Source: CAD feature listing. Evaluate the final solid. Frame: model axes, mm. A direction names the side the tool comes from. Give positions to 0.01 mm unless a question says otherwise; leave off trailing zeros. Write each loop counter-clockwise with the first axis right and the second up, starting at its lowest first coordinate (ties: lowest second). Pieces come first, ordered by that corner, then holes. Notation, with made-up numbers: M -20.75,36.5 L 38.25,36.5 A30 cw 38.25,71.5 Z; hole C -9.75,69 d10. An arc over 180 degrees is marked long. Answer as a JSON object with one key per item and string values. Group by question number.
```python
from build123d import *

# Parameters (mm, degrees)
SKETCH1_R           = 1.6
BOSS_EXTRUDE1_DEPTH = 2.5
SKETCH2_W           = 66
SKETCH2_H           = 2.5
BOSS_EXTRUDE2_DEPTH = 43
SKETCH3_W           = 5
SKETCH3_H           = 32.5
CUT_EXTRUDE1_DEPTH  = 9.5
LPATTERN1_COUNT     = 6
LPATTERN1_PITCH     = 10
SKETCH4_W           = 4
SKETCH4_H           = 15
CUT_EXTRUDE2_DEPTH  = 44
LPATTERN2_COUNT     = 5
LPATTERN2_PITCH     = 8


with BuildPart() as part:
    # Sketch1 → Boss-Extrude1 (new body)
    with BuildSketch(Plane(origin=(0, 0, 0), x_dir=(1, 0, 0), z_dir=(0, 1, 0))):
        Polygon((-33, 6), (-33, 16), (33, 16), (33, 6), (33, -6), (-33, -6), align=None)
        with Locations((-26, 11)):
            Circle(SKETCH1_R, mode=Mode.SUBTRACT)
        with Locations((-14.5, 11)):
            Circle(SKETCH1_R, mode=Mode.SUBTRACT)
    extrude(amount=BOSS_EXTRUDE1_DEPTH)

    # Sketch2 → Boss-Extrude2 (add)
    with BuildSketch(Plane(origin=(0, 0, 0), x_dir=(1, 0, 0), z_dir=(0, 1, 0))):
        with Locations((0, -7.25)):
            Rectangle(SKETCH2_W, SKETCH2_H)
    extrude(amount=BOSS_EXTRUDE2_DEPTH)

    # Sketch3 → Cut-Extrude1 (cut, through all)
    with BuildSketch(Plane.XY):
        with Locations((25.5, 22.75)):
            Rectangle(SKETCH3_W, SKETCH3_H)
    cut_extrude1 = extrude(amount=CUT_EXTRUDE1_DEPTH, mode=Mode.SUBTRACT)

    # LPattern1: Cut-Extrude1 ×6
    with Locations(*[(-i * LPATTERN1_PITCH, 0, 0) for i in range(1, LPATTERN1_COUNT)]):
        add(cut_extrude1, mode=Mode.SUBTRACT)

    # Sketch4 → Cut-Extrude2 (cut, through all)
    with BuildSketch(Plane(origin=(0, 0, 0), x_dir=(1, 0, 0), z_dir=(0, 1, 0))):
        with Locations((26, 5)):
            Rectangle(SKETCH4_W, SKETCH4_H)
    cut_extrude2 = extrude(amount=CUT_EXTRUDE2_DEPTH, mode=Mode.SUBTRACT)

    # LPattern2: Cut-Extrude2 ×5
    with Locations(*[(-i * LPATTERN2_PITCH, 0, 0) for i in range(1, LPATTERN2_COUNT)]):
        add(cut_extrude2, mode=Mode.SUBTRACT)


solid = part.part
```
(1) Section D-D, the plane z = -6. Return loops of the section in (x, y), plus the area to 3 significant figures.
(2) Ray query, L1, parallel to Z at x = -26, y = 0.9; L2, parallel to Y at x = 22, z = 3.25; L3, parallel to Z at x = 1, y = 9. Return the intervals inside material, ascending. Write a range as [from, to].
(3) Pull-direction query (Y, two-part tool) for faces 1 (the flat face through (2, 1, -12.5)), 2 (the flat face through (-0.5, 0, -3.9)), 3 (the flat face through (7.8, 2.5, -5.2)), 4 (the flat face through (28, 23, 7)); classes: pulls with the +Y half, pulls with the -Y half, needs draft (parallel to the pull), parting line crosses it, or undercut.
(4) Contact query for a flat-ended pin moving along its axis: pin 1 Ø12 at (x, z) = (8, -10) entering from +Y. Output: stop coordinate, or through.
(5) Section B-B, the plane y = 17. Return loops of the section in (x, z).
(6) Section C-C, the plane x = -14.5. Return loops of the section in (y, z).
(7) Access query for faces 5 (the flat face through (-33, 15, 6.3)), 6 (the flat face through (25, 39, 7)), 7 (the flat face through (10, 1, -12.5)). Directions: +Z, -Z, +X, -X, +Y, -Y. A direction counts if a zero-diameter tool reaches every point of the face in a straight line with its end or side. Return the directions, or none.
(8) Section A-A, the plane z = -11. State how many separate pieces and enclosed holes the cut face has, plus the area to 3 significant figures.
Reported:
{
 "1": {"outline": "M -33,0 L -8,0 L -8,2.5 L -33,2.5 Z; M -4,0 L 0,0 L 0,2.5 L -4,2.5 Z; M 4,0 L 8,0 L 8,2.5 L 4,2.5 Z; M 12,0 L 16,0 L 16,2.5 L 12,2.5 Z; M 20,0 L 24,0 L 24,2.5 L 20,2.5 Z; M 28,0 L 33,0 L 33,2.5 L 28,2.5 Z", "area": "115 mm2"},
 "2": {"L1": "z = [-16, -12.6], [-9.4, 8.5]", "L2": "y = [0, 2.5]", "L3": "z = [6, 8.5]"},
 "3": {"face 1": "needs draft", "face 2": "pulls with the -Y half", "face 3": "pulls with the +Y half", "face 4": "undercut"},
 "4": {"pin 1": "stops at y = 2.5"},
 "5": {"outline": "M -33,6 L -27,6 L -27,8.5 L -33,8.5 Z; M -22,6 L -17,6 L -17,8.5 L -22,8.5 Z; M -12,6 L -7,6 L -7,8.5 L -12,8.5 Z; M -2,6 L 3,6 L 3,8.5 L -2,8.5 Z; M 8,6 L 13,6 L 13,8.5 L 8,8.5 Z; M 18,6 L 23,6 L 23,8.5 L 18,8.5 Z; M 28,6 L 33,6 L 33,8.5 L 28,8.5 Z"},
 "6": {"outline": "M 0,-16 L 2.5,-16 L 2.5,-12.6 L 0,-12.6 Z; M 0,-9.4 L 2.5,-9.4 L 2.5,6 L 6.5,6 L 6.5,8.5 L 0,8.5 Z; M 39,6 L 43,6 L 43,8.5 L 39,8.5 Z"},
 "7": {"face 5": "+Z, -Z, -X, +Y, -Y", "face 6": "+Z, -Z", "face 7": "+Y, -Y"},
 "8": {"separate pieces": "8", "enclosed holes": "0", "area": "99.0 mm2"}
}
